Autodesk Inventor part; units mm, degrees
ref_plane "YZ Plane" through (0, 0, 0) normal (1, 0, 0) x (0, 1, 0)
ref_plane "XZ Plane" through (0, 0, 0) normal (0, 1, 0) x (-1, 0, 0)
ref_plane "XY Plane" through (0, 0, 0) normal (0, 0, 1) x (1, 0, 0)
sketch "Sketch1" plane through (0, 0, 0) normal (0, 1, 0) x (-1, 0, 0)
  arc A0 (-166.5, -1.5) -> (-165, 0) centre (-166.5, 0) ccw
  line L0 (-165, 0) -> (-158, 0)
  arc A1 (-158, 0) -> (-156.5, 1.5) centre (-158, 1.5) ccw
  line L1 (-156.5, 1.5) -> (-156.5, 10)
  line L2 (-156.5, 10) -> (-138.6622, 12.2297)
  arc A2 (-134.321, 12.5) -> (-138.6622, 12.2297) centre (-134.321, -22.5) ccw
  line L3 (-134.321, 12.5) -> (-23.3333, 12.5)
  arc A3 (-23.3333, 12.5) -> (-17.3333, 14.5) centre (-23.3333, 22.5) ccw
  line L4 (-17.3333, 14.5) -> (-12.6667, 18)
  arc A4 (-6.6667, 20) -> (-12.6667, 18) centre (-6.6667, 10) ccw
  line L5 (-6.6667, 20) -> (5.4953, 20)
  arc A5 (12.9849, 16.6262) -> (5.4953, 20) centre (5.4953, 10) ccw
  line L6 (12.9849, 16.6262) -> (21.8321, 6.6262)
  arc A6 (21.8321, -6.6262) -> (21.8321, 6.6262) centre (14.3426, 0) ccw
  line L7 (21.8321, -6.6262) -> (12.9849, -16.6262)
  arc A7 (5.4953, -20) -> (12.9849, -16.6262) centre (5.4953, -10) ccw
  line L8 (5.4953, -20) -> (-6.6667, -20)
  arc A8 (-12.6667, -18) -> (-6.6667, -20) centre (-6.6667, -10) ccw
  line L9 (-12.6667, -18) -> (-17.3333, -14.5)
  arc A9 (-17.3333, -14.5) -> (-23.3333, -12.5) centre (-23.3333, -22.5) ccw
  line L10 (-23.3333, -12.5) -> (-134.321, -12.5)
  arc A10 (-138.6622, -12.2297) -> (-134.321, -12.5) centre (-134.321, 22.5) ccw
  line L11 (-138.6622, -12.2297) -> (-156.5, -10)
  line L12 (-156.5, -10) -> (-165, -10)
  arc A11 (-166.5, -8.5) -> (-165, -10) centre (-165, -8.5) ccw
  line L13 (-166.5, -8.5) -> (-166.5, -1.5)
  arc A12 (4.5962, 6.7175) -> (6.7175, 4.5962) centre (5.6569, 5.6569) ccw
  line L14 (6.7175, 4.5962) -> (7.7782, 5.6569)
  arc A13 (7.7782, 5.6569) -> (5.6569, 7.7782) centre (6.7175, 6.7175) ccw
  line L15 (5.6569, 7.7782) -> (4.5962, 6.7175)
  line L16 (-4.5962, -6.7175) -> (-5.6569, -7.7782)
  arc A14 (-7.7782, -5.6569) -> (-5.6569, -7.7782) centre (-6.7175, -6.7175) ccw
  line L17 (-7.7782, -5.6569) -> (-6.7175, -4.5962)
  arc A15 (-4.5962, -6.7175) -> (-6.7175, -4.5962) centre (-5.6569, -5.6569) ccw
  arc A16 (6.7175, -4.5962) -> (4.5962, -6.7175) centre (5.6569, -5.6569) ccw
  line L18 (4.5962, -6.7175) -> (5.6569, -7.7782)
  arc A17 (5.6569, -7.7782) -> (7.7782, -5.6569) centre (6.7175, -6.7175) ccw
  line L19 (7.7782, -5.6569) -> (6.7175, -4.5962)
  line L20 (-5.6569, 7.7782) -> (-4.5962, 6.7175)
  arc A18 (-6.7175, 4.5962) -> (-4.5962, 6.7175) centre (-5.6569, 5.6569) ccw
  line L21 (-6.7175, 4.5962) -> (-7.7782, 5.6569)
  arc A19 (-5.6569, 7.7782) -> (-7.7782, 5.6569) centre (-6.7175, 6.7175) ccw
  circle A20 centre (-136.5, -6) radius 1.5
  circle A21 centre (-124.0736, 0) radius 1.5
  circle A22 centre (-144.9332, 0) radius 4
  circle A23 centre (0, 0) radius 3
  circle A24 centre (-136.5, 6) radius 1.5
  point P0 (5.4953, -20)
  point P1 (12.9849, -16.6262)
  point P2 (21.8321, -6.6262)
  point P3 (21.8321, 6.6262)
  point P4 (-12.6667, 18)
  point P5 (-165, -10)
  point P6 (7.7782, 5.6569)
  point P7 (5.6569, 7.7782)
  point P8 (6.7175, -4.5962)
  point P9 (5.6569, -7.7782)
  point P10 (4.5962, -6.7175)
  point P11 (-4.5962, -6.7175)
  point P12 (-5.6569, -7.7782)
  point P13 (-6.7175, -4.5962)
  point P14 (-7.7782, 5.6569)
  point P15 (-5.6569, 7.7782)
extrude "Extrusion1" add sketch "Sketch1" along normal blind 6
properties part number "TokerCNC arm"
Design review of the part built by this model. Coordinates are the model's own, in mm. A direction names the side the tool comes from. Coordinates: 2 decimals unless noted, no trailing zeros. Loops run counter-clockwise (first coordinate to the right, second up) from the corner with the lowest first, then second, coordinate; pieces in that order, holes last.
Item 1: Clearance check with flat-ended pins moving along their axes: pin 1 (3 mm diameter, centred on x = 17.5, y = 2, fed in from +Z); pin 2 (1.8 mm diameter, centred on x = 68, y = 2, fed in from -Z); pin 3 (1.8 mm diameter, centred on x = 161.5, y = 1.5, fed in from +Z). State where each tip first meets the part, or that it passes through.
Completed:
pin 1: stops at z = 15.5
pin 2: stops at z = -12.5
pin 3: stops at z = 0
Item 2: Wall thickness on L1, parallel to Z at x = -7, y = 0.6; L2, parallel to Z at x = 136.5, y = 1.35; L3, parallel to X at y = 4.3, z = 7: over which ranges is each line inside the solid? List them lowest first.
Completed:
L1: z = -19.89 to -8.19, -4.88 to 4.88, 8.19 to 19.89
L2: z = -12.43 to -7.5, -4.5 to 4.5, 7.5 to 12.43
L3: x = -21.5 to -8.19, -4.88 to 4.88, 8.19 to 135.38, 137.62 to 156.5
Item 3: Add section A-A (y = 2.5). Give the number of separate pieces and of enclosed holes in the cut face, and give its area (3 significant figures).
Completed:
separate pieces: 1
enclosed holes: 9
area: 4,770 mm2
Item 4: Draft analysis for pull direction Z (two halves, no side actions). For faces 1 (the flat face through (51, 6, 0)), 2 (the cylindrical face through (122.643, 2.958, -0.451)), 3 (the cylindrical face through (-9.66, 2.96, -19.09)), 4 (the cylindrical face through (3, 3, 0)), state which applies: pulls with the +Z half, pulls with the -Z half, needs draft (parallel to the pull), parting line crosses it, or undercut.
Completed:
face 1: needs draft
face 2: undercut
face 3: pulls with the -Z half
face 4: undercut
Item 5: Add section B-B (x = 44). Write out the cut boundary in (y, z).
Completed:
outline: (0, -12.5) - (6, -12.5) - (6, 12.5) - (0, 12.5) - close
Item 6: For faces 5 (the flat face through (78, 3, -12.5)), 6 (the flat face through (162, 3, 0)), 7 (the cylindrical face through (-9.55, 2.96, 19.14)), list the 3-axis set-ups (+Z, -Z, +X, -X, +Y, -Y) from which the entire face can be reached by the end or side of a thin tool; tool diameter is ignored.
Completed:
face 5: -Z, +X, +Y, -Y
face 6: +Z, +X, +Y, -Y
face 7: +Z, -X, +Y, -Y
